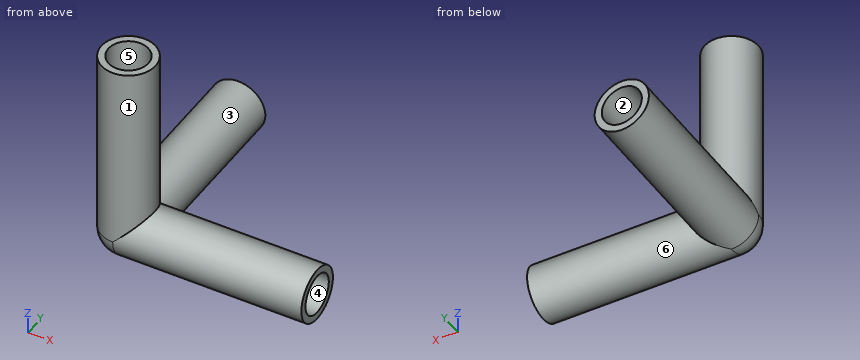
```python
from build123d import *

# Parameters (mm, degrees)
SKETCH_1_R      = 5.75
SKETCH_1_R_2    = 4.25
EXTRUDE_1_DEPTH = 40
SKETCH_2_R      = 5.75
SKETCH_2_R_2    = 4.25
EXTRUDE_2_DEPTH = 40
SKETCH_3_R      = 5.75
SKETCH_3_R_2    = 4.25
EXTRUDE_3_DEPTH = 40


with BuildPart() as part:
    # 草图1 → 凸台-拉伸1 (new body)
    with BuildSketch(Plane.XY):
        Circle(SKETCH_1_R)
        Circle(SKETCH_1_R_2, mode=Mode.SUBTRACT)
    extrude(amount=EXTRUDE_1_DEPTH)

    # 草图2 → 凸台-拉伸2 (add)
    with BuildSketch(Plane(origin=(0, 0, 0), x_dir=(1, 0, 0), z_dir=(0, 1, 0))):
        with Locations(Location((0, 0, 0), (0, 0, 180))):
            Circle(SKETCH_2_R)
        Circle(SKETCH_2_R_2, mode=Mode.SUBTRACT)
    extrude(amount=EXTRUDE_2_DEPTH)

    # 草图3 → 凸台-拉伸3 (add)
    with BuildSketch(Plane(origin=(0, 0, 0), x_dir=(0, 0, -1), z_dir=(1, 0, 0))):
        Circle(SKETCH_3_R)
        Circle(SKETCH_3_R_2, mode=Mode.SUBTRACT)
    extrude(amount=EXTRUDE_3_DEPTH)

    # 草图4 → 旋转1 (revolve)
    with BuildSketch(Plane(origin=(0, 0, 0), x_dir=(-1, 0, 0), z_dir=(0, 0, -1)), mode=Mode.PRIVATE) as revolve_1_sk:
        with BuildLine():
            Line((4.25, 0), (5.75, 0))
            ThreePointArc((5.75, 0), (4.065863992, -4.065863992), (0, -5.75))
            Line((0, -5.75), (0, -4.25))
            ThreePointArc((0, -4.25), (3.00520382, -3.00520382), (4.25, 0))
        make_face()
    revolve(revolve_1_sk.sketch.rotate(Axis((0, -4.25, 0), (0, 1, 0)), 270), axis=Axis((0, -4.25, 0), (0, 1, 0)))


solid = part.part
```
Could you check a few things on this model? Use its own coordinates, in mm. Face numbers are marked on the shaded views. A direction names the side the tool comes from. Coordinates: 2 decimals unless noted, no trailing zeros. Order: outer loops, then holes, each group sorted by start corner. A loop starts at its lowest first (then second) coordinate and runs counter-clockwise, first axis right, second up. Notation, with made-up numbers: M -24,55.25 L 20,55.25 A23 ccw 20,88.25 Z; hole C -23,52.5 d9. An arc over 180 degrees is marked long. Use a Markdown table: item, result. Add a question column.
Q1. We'd pull the mould along Y, two halves only. Please class the marked faces 3, 4, 5 and 6: pulls with the +Y half, pulls with the -Y half, needs draft (parallel to the pull), parting line crosses it, or undercut.
Q2. I want a section at A-A on z = 26. List the corners of the cut face in (x, y) for me.
Q3. Which directions (+Z, -Z, +X, -X, +Y, -Y) give clear straight access to the entire face, cutting with the end or side of a thin tool? Please do the marked faces 1 and 2.
Q4. If I drill on L1, parallel to X at y = 21, z = 0, over which ranges is the centre line in solid material (lowest first)?
Q5. I want a section at C-C on x = -2. List the corners of the cut face in (y, z) for me.
Q6. I'm going to push flat-ended pins straight in: pin 1 (1.3 mm diameter, centred on y = 3.5, z = -3, fed in from -X); pin 2 (1.3 mm diameter, centred on x = -2, y = 3.5, fed in from -Z); pin 3 (7.5 mm diameter, centred on x = 0, y = 0, fed in from +Z); pin 4 (10 mm diameter, centred on x = 0, z = 0, fed in from +Y). Where does each tip first touch, or does it pass through?
Checked values:
| question | item | result |
|---|---|---|
| 1 | face 3 | needs draft |
| 1 | face 4 | undercut |
| 1 | face 5 | undercut |
| 1 | face 6 | parting line crosses it |
| 2 | outline | C 0,0 d11.5; hole C 0,0 d8.5 |
| 3 | face 1 | +Z |
| 3 | face 2 | +Y |
| 4 | L1 | -5.75 to -4.25, 4.25 to 5.75 |
| 5 | outline | M -5.39,0 A5.39 ccw 0,-5.39 L 40,-5.39 L 40,-3.75 L 0,-3.75 A3.75 cw 0,3.75 L 3.75,3.75 L 3.75,0 L 5.39,0 L 5.39,3.75 L 40,3.75 L 40,5.39 L 5.39,5.39 L 5.39,40 L 3.75,40 L 3.75,5.39 L 0,5.39 A5.39 ccw -3.75,3.87 L -3.75,40 L -5.39,40 Z |
| 6 | pin 1 | x = -5.25 |
| 6 | pin 2 | z = -5.59 |
| 6 | pin 3 | z = 5.75 |
| 6 | pin 4 | y = 40 |
